Geometry: final body of the model. Coordinates: model frame, mm. Give positions to 0.01 mm unless a question says otherwise; leave off trailing zeros. Write each loop counter-clockwise with the first axis right and the second up, starting at its lowest first coordinate (ties: lowest second). Pieces come first, ordered by that corner, then holes.
Q1. Section B-B (y = -49). Return the cut outline in (x, z), plus the area to 3 significant figures.
Q2. Section A-A (x = 53). Return the cut outline in (y, z).
Q3. Line query: line 1 (Y direction, x = -4.5, z = 3.75); line 2 (X direction, y = -158.5, z = 3.5). Output: solid intervals per line, ascending.
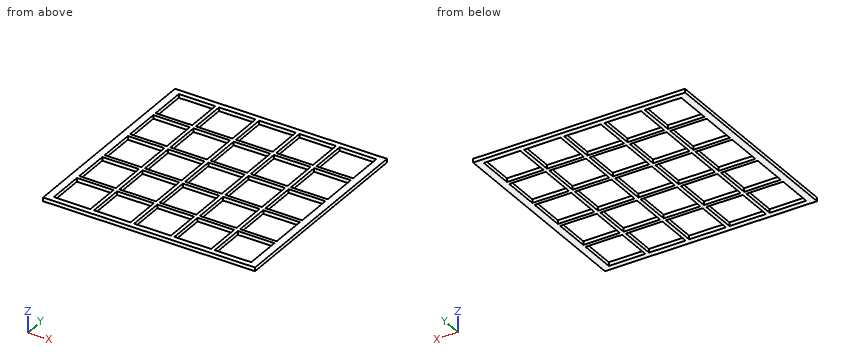
from build123d import *

# Parameters (mm, degrees)
F0_W     = 368.3
F0_H     = 361.95
F0_W_2   = 63.5
F0_H_2   = 63.5
F1_DEPTH = 6.35


with BuildPart() as f1:
    # F0 (on Top) → F1 (new body)
    with BuildSketch(Plane.XY):
        with Locations((9.59555, 5.294811)):
            Rectangle(F0_W, F0_H)
        with Locations((-130.10445, -134.405189)):
            Rectangle(F0_W_2, F0_H_2, mode=Mode.SUBTRACT)
        with Locations((-60.25445, -134.405189)):
            Rectangle(F0_W_2, F0_H_2, mode=Mode.SUBTRACT)
        with Locations((-130.10445, -64.555189)):
            Rectangle(F0_W_2, F0_H_2, mode=Mode.SUBTRACT)
        with Locations((-130.10445, 5.294811)):
            Rectangle(F0_W_2, F0_H_2, mode=Mode.SUBTRACT)
        with Locations((-60.25445, -64.555189)):
            Rectangle(F0_W_2, F0_H_2, mode=Mode.SUBTRACT)
        with Locations((-60.25445, 5.294811)):
            Rectangle(F0_W_2, F0_H_2, mode=Mode.SUBTRACT)
        with Locations((9.59555, -134.405189)):
            Rectangle(F0_W_2, F0_H_2, mode=Mode.SUBTRACT)
        with Locations((79.44555, -134.405189)):
            Rectangle(F0_W_2, F0_H_2, mode=Mode.SUBTRACT)
        with Locations((149.29555, -134.405189)):
            Rectangle(F0_W_2, F0_H_2, mode=Mode.SUBTRACT)
        with Locations((9.59555, -64.555189)):
            Rectangle(F0_W_2, F0_H_2, mode=Mode.SUBTRACT)
        with Locations((79.44555, -64.555189)):
            Rectangle(F0_W_2, F0_H_2, mode=Mode.SUBTRACT)
        with Locations((9.59555, 5.294811)):
            Rectangle(F0_W_2, F0_H_2, mode=Mode.SUBTRACT)
        with Locations((79.44555, 5.294811)):
            Rectangle(F0_W_2, F0_H_2, mode=Mode.SUBTRACT)
        with Locations((149.29555, -64.555189)):
            Rectangle(F0_W_2, F0_H_2, mode=Mode.SUBTRACT)
        with Locations((149.29555, 5.294811)):
            Rectangle(F0_W_2, F0_H_2, mode=Mode.SUBTRACT)
        with Locations((-130.10445, 75.144811)):
            Rectangle(F0_W_2, F0_H_2, mode=Mode.SUBTRACT)
        with Locations((-60.25445, 75.144811)):
            Rectangle(F0_W_2, F0_H_2, mode=Mode.SUBTRACT)
        with Locations((-130.10445, 144.994811)):
            Rectangle(F0_W_2, F0_H_2, mode=Mode.SUBTRACT)
        with Locations((-60.25445, 144.994811)):
            Rectangle(F0_W_2, F0_H_2, mode=Mode.SUBTRACT)
        with Locations((9.59555, 75.144811)):
            Rectangle(F0_W_2, F0_H_2, mode=Mode.SUBTRACT)
        with Locations((79.44555, 75.144811)):
            Rectangle(F0_W_2, F0_H_2, mode=Mode.SUBTRACT)
        with Locations((149.29555, 75.144811)):
            Rectangle(F0_W_2, F0_H_2, mode=Mode.SUBTRACT)
        with Locations((9.59555, 144.994811)):
            Rectangle(F0_W_2, F0_H_2, mode=Mode.SUBTRACT)
        with Locations((79.44555, 144.994811)):
            Rectangle(F0_W_2, F0_H_2, mode=Mode.SUBTRACT)
        with Locations((149.29555, 144.994811)):
            Rectangle(F0_W_2, F0_H_2, mode=Mode.SUBTRACT)
    extrude(amount=F1_DEPTH)


solid = f1.part
Computed:
1. outline: (-174.55, 0) - (-161.85, 0) - (-161.85, 6.35) - (-174.55, 6.35) - close; (-98.35, 0) - (-92, 0) - (-92, 6.35) - (-98.35, 6.35) - close; (-28.5, 0) - (-22.15, 0) - (-22.15, 6.35) - (-28.5, 6.35) - close; (41.35, 0) - (47.7, 0) - (47.7, 6.35) - (41.35, 6.35) - close; (111.2, 0) - (117.55, 0) - (117.55, 6.35) - (111.2, 6.35) - close; (181.05, 0) - (193.75, 0) - (193.75, 6.35) - (181.05, 6.35) - close
1. area: 323 mm2
2. outline: (-175.68, 0) - (-166.16, 0) - (-166.16, 6.35) - (-175.68, 6.35) - close; (-102.66, 0) - (-96.31, 0) - (-96.31, 6.35) - (-102.66, 6.35) - close; (-32.81, 0) - (-26.46, 0) - (-26.46, 6.35) - (-32.81, 6.35) - close; (37.04, 0) - (43.39, 0) - (43.39, 6.35) - (37.04, 6.35) - close; (106.89, 0) - (113.24, 0) - (113.24, 6.35) - (106.89, 6.35) - close; (176.74, 0) - (186.27, 0) - (186.27, 6.35) - (176.74, 6.35) - close
3. line 1: y = -175.68 to -166.16, -102.66 to -96.31, -32.81 to -26.46, 37.04 to 43.39, 106.89 to 113.24, 176.74 to 186.27
3. line 2: x = -174.55 to -161.85, -98.35 to -92, -28.5 to -22.15, 41.35 to 47.7, 111.2 to 117.55, 181.05 to 193.75
